Autodesk Inventor part; units mm, degrees
ref_plane "Work Plane1" through (0, 6.35, 0) normal (0, 1, 0) x (-1, 0, 0)
ref_plane "YZ Plane" through (0, 0, 0) normal (1, 0, 0) x (0, 1, 0)
ref_plane "XY Plane" through (0, 0, 0) normal (0, 0, 1) x (1, 0, 0)
sketch "Sketch1" plane through (0, 0, 0) normal (0, 0, 1) x (1, 0, 0)
  circle A0 centre (0, 0) radius 6.35
  dimension "d0" = 12.7
extrude "Extrusion1" add sketch "Sketch1" along normal blind 660.4
sketch "Sketch2" plane through (0, 0, 660.4) normal (0, 0, 1) x (1, 0, 0)
  circle A0 centre (0, 0) radius 5.334
  dimension "d3" = 10.668
extrude "Extrusion2" cut sketch "Sketch2" against normal blind 660.4
ref_plane "Work Plane1" through (0, 6.35, 0) normal (0, 1, 0) x (-1, 0, 0)
sketch "Sketch3" plane through (0, 6.35, 0) normal (0, 1, 0) x (-1, 0, 0)
  circle A0 centre (0, 330.2) radius 2.8654
  point P0 (0, 0)
  dimension "d6" = 330.2
extrude "Extrusion3" cut sketch "Sketch3" against normal through all
properties part number "horizontal support"
Geometry check sheet. Reference: the model listing, model coordinates, mm. Round coordinates to 2 decimals unless told otherwise and drop trailing zeros. Write each loop counter-clockwise with the first axis right and the second up, starting at its lowest first coordinate (ties: lowest second). Pieces come first, ordered by that corner, then holes. Notation, with made-up numbers: (-39.5, 82.5) - (8.5, 82.5) arc R14 ccw to (8.5, 108.5) - close; hole circle Ø1 at (-24.5, 6.5). An arc over 180 degrees is marked (long way). One line per item, written item: value.
1. Cross-section at A-A on x = 0. Record the boundary of the cut face in (y, z), and give its area (3 significant figures).
The answers:
outline: (-6.35, 0) - (-5.33, 0) - (-5.33, 327.33) - (-6.35, 327.33) - close; (-6.35, 333.07) - (-5.33, 333.07) - (-5.33, 660.4) - (-6.35, 660.4) - close; (5.33, 0) - (6.35, 0) - (6.35, 327.33) - (5.33, 327.33) - close; (5.33, 333.07) - (6.35, 333.07) - (6.35, 660.4) - (5.33, 660.4) - close
area: 1,330 mm^2
2. Mould release check, pull along Y, two halves, no side actions. Record for faces 1 (the face through (2.461, -4.732, 334.823)), 2 (the face through (-1.38, 6.2, 325.58)): released by +Y, released by -Y, zero draft, split by the parting line, or undercut.
The answers:
face 1: undercut
face 2: split by the parting line
3. Cross-section at C-C on z = 377. Record the boundary of the cut face in (x, y), and give its area (3 significant figures).
The answers:
outline: circle Ø12.7 at (0, 0); hole circle Ø10.67 at (0, 0)
area: 37.3 mm^2
4. Cross-section at B-B on y = 0. Record the boundary of the cut face in (x, z), and give its area (3 significant figures).
The answers:
outline: (-6.35, 0) - (-5.33, 0) - (-5.33, 660.4) - (-6.35, 660.4) - close; (5.33, 0) - (6.35, 0) - (6.35, 660.4) - (5.33, 660.4) - close
area: 1,340 mm^2
5. Depth check by flat-ended pin: pin 1 Ø1 at (x, z) = (-2.5, 395) entering from -Y; pin 2 Ø4 at (y, z) = (-4.5, 384.5) entering from -X; pin 3 Ø1 at (x, z) = (-5, 160.5) entering from -Y. Enter the tip coordinate at first touch or a pass-through.
The answers:
pin 1: stops at y = -6.03
pin 2: stops at x = -5.84
pin 3: stops at y = -4.48
6. Scan lines: L1, parallel to Y at x = 0, z = 323; L2, parallel to Z at x = 0, y = -5.7; L3, parallel to X at y = -4.5, z = 521. Record each from-to range of solid material in increasing order.
The answers:
L1: y = -6.35 to -5.33, 5.33 to 6.35
L2: z = 0 to 327.33, 333.07 to 660.4
L3: x = -4.48 to -2.86, 2.86 to 4.48
